Could you check a few things on this model? Use its own coordinates, in mm. A direction names the side the tool comes from. Coordinates: 2 decimals unless noted, no trailing zeros. Loops run counter-clockwise (first coordinate to the right, second up) from the corner with the lowest first, then second, coordinate; pieces in that order, holes last.
1) Imagine slicing it at A-A on x = 23.5. Please give me the cut outline in (y, z).
2) Thinking about a two-plate mould opening in Y: for faces 3 (the face through (0.43, 0.45, 0.51)), 4 (the face through (0, 23.2, 0.5)), 5 (the face through (8.5, 23.3, 0.5)), which applies, released by +Y, released by -Y, zero draft, split by the parting line, or undercut?
3) Will this pin go through, and if not, where does the flat tip stop? P1, Ø1.5, axis at x = 37.5, y = 11.5, coming from the -Z side.
4) If I drill on line 1 along Y through (x, z) = (23.5, 0.3); line 2 along Y through (x, z) = (31, 0.1); line 3 along Y through (x, z) = (42.25, 0.4), over which ranges is the centre line in solid material (lowest first)?
5) For faces 1 (the face through (23.3, 8.5, 0.5)), 2 (the face through (23.2, 0, 0.5)), which set-ups out of +Z, -Z, +X, -X, +Y, -Y let a thin tool reach every point of the face, with its end or its side?
6) Imagine slicing it at B-B on y = 25. Please give me the cut outline in (x, z), plus the area to 3 significant figures.
7) Imagine slicing it at C-C on x = 34.5. Please give me the cut outline in (y, z), plus the area to 3 significant figures.
```python
from build123d import *

# Parameters (mm, degrees)
SKETCH1_W           = 47
SKETCH1_H           = 47
SKETCH1_R           = 2.5
SKETCH1_W_2         = 30
SKETCH1_H_2         = 30
BOSS_EXTRUDE1_DEPTH = 1
FILLET1_R           = 1.5


with BuildPart() as part:
    # Sketch1 → Boss-Extrude1 (new body)
    with BuildSketch(Plane.XY):
        with Locations((23.5, 23.5)):
            Rectangle(SKETCH1_W, SKETCH1_H)
        with Locations((23.5, 4.75)):
            Circle(SKETCH1_R, mode=Mode.SUBTRACT)
        with Locations((42.25, 23.5)):
            Circle(SKETCH1_R, mode=Mode.SUBTRACT)
        with Locations((23.5, 42.25)):
            Circle(SKETCH1_R, mode=Mode.SUBTRACT)
        with Locations((4.75, 23.5)):
            Circle(SKETCH1_R, mode=Mode.SUBTRACT)
        with Locations((23.5, 23.5)):
            Rectangle(SKETCH1_W_2, SKETCH1_H_2, mode=Mode.SUBTRACT)
    extrude(amount=BOSS_EXTRUDE1_DEPTH)

    # Fillet1
    fillet1_edges = [part.edges().sort_by_distance(p)[0] for p in [
        (0, 47, 0.5),
        (47, 47, 0.5),
        (47, 0, 0.5),
        (0, 0, 0.5),
    ]]
    fillet(fillet1_edges, radius=FILLET1_R)


solid = part.part
```
Filled in:
1. outline: (0, 0) - (2.25, 0) - (2.25, 1) - (0, 1) - close; (7.25, 0) - (8.5, 0) - (8.5, 1) - (7.25, 1) - close; (38.5, 0) - (39.75, 0) - (39.75, 1) - (38.5, 1) - close; (44.75, 0) - (47, 0) - (47, 1) - (44.75, 1) - close
2. face 3: released by -Y
2. face 4: zero draft
2. face 5: undercut
3. P1: passes through
4. line 1: y = 0 to 2.25, 7.25 to 8.5, 38.5 to 39.75, 44.75 to 47
4. line 2: y = 0 to 8.5, 38.5 to 47
4. line 3: y = 0 to 21, 26 to 47
5. face 1: +Z, -Z
5. face 2: +Z, -Z, +X, -X, -Y
6. outline: (0, 0) - (2.75, 0) - (2.75, 1) - (0, 1) - close; (6.75, 0) - (8.5, 0) - (8.5, 1) - (6.75, 1) - close; (38.5, 0) - (40.25, 0) - (40.25, 1) - (38.5, 1) - close; (44.25, 0) - (47, 0) - (47, 1) - (44.25, 1) - close
6. area: 9.00 mm2
7. outline: (0, 0) - (8.5, 0) - (8.5, 1) - (0, 1) - close; (38.5, 0) - (47, 0) - (47, 1) - (38.5, 1) - close
7. area: 17.0 mm2
